```python
from build123d import *

# Parameters (mm, degrees)
SKETCH1_W           = 100
SKETCH1_H           = 6.794919243
BOSS_EXTRUDE1_DEPTH = 102.5
CIRPATTERN1_COUNT   = 4


with BuildPart() as part:
    # Sketch1 → Boss-Extrude1 (new, symmetric)
    with BuildSketch(Plane(origin=(0, 0, 0), x_dir=(0, 0, -1), z_dir=(1, 0, 0))):
        Polygon((-200, 0), (-100, 0), (-100, 6.794919243), (-100, 26.794919243), align=None)
        with Locations((-50, 3.397459622)):
            Rectangle(SKETCH1_W, SKETCH1_H)
    boss_extrude1 = extrude(amount=BOSS_EXTRUDE1_DEPTH, both=True)

    # CirPattern1: Boss-Extrude1 ×4 about axis
    cirpattern1_axis = Axis((0, 0, 0), (0, 1, 0))
    for i in range(1, CIRPATTERN1_COUNT):
        add(boss_extrude1.rotate(cirpattern1_axis, i * 360 / CIRPATTERN1_COUNT))


solid = part.part
```
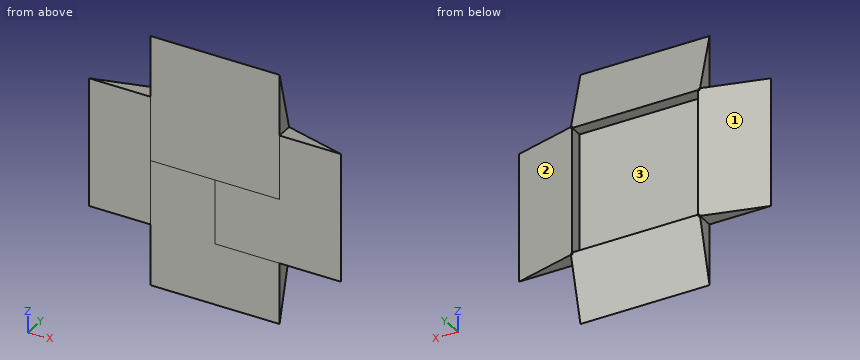
Could you check a few things on this model? Use its own coordinates, in mm. Face numbers are marked on the shaded views. Give positions to 0.01 mm unless a question says otherwise; leave off trailing zeros. Write each loop counter-clockwise with the first axis right and the second up, starting at its lowest first coordinate (ties: lowest second). Pieces come first, ordered by that corner, then holes. Notation, with made-up numbers: (8.25, 45) - (14.25, 45) arc R28 ccw to (14.25, 65) - close; hole circle Ø9 at (26.25, -3.5). An arc over 180 degrees is marked (long way). One line per item, written item: value. Start each with the question number.
Item 1: Imagine slicing it at D-D, the plane x = -152. List the corners of the cut face in (y, z) for me, and give its area (3 significant figures).
Item 2: I'm going to push flat-ended pins straight in: pin 1 (8 mm diameter, centred on x = -171, y = 15, fed in from -Z); pin 2 (5 mm diameter, centred on x = -115.5, y = 12.5, fed in from -Z); pin 3 (4 mm diameter, centred on x = 33.5, z = 80, fed in from +Y); pin 4 (13 mm diameter, centred on x = -145, y = 7.5, fed in from +Z). Where does each tip first touch, or does it pass through?
Item 3: Imagine slicing it at C-C, the plane y = 12.5. List the corners of the cut face in (x, z) for me, and give its area (3 significant figures).
Item 4: If we mould it in two halves opening along X, with no side actions, what happens to the marked faces 1, 2 and 3? For each: +X half, -X half, draft (parallel to the pull), parting line (faces both ways), or undercut.
Item 5: Imagine slicing it at A-A, the plane z = 76.5. List the corners of the cut face in (x, y) for me, and give its area (3 significant figures).
Item 6: Please list where these lines run through material, in increasing order: line 1 (Y direction, x = -47.5, z = 76.5); line 2 (X direction, y = 1, z = -141.5). Write a range as from..to.
Item 7: Imagine slicing it at B-B, the plane x = 54. List the corners of the cut face in (y, z) for me.
Geometry says:
1. outline: (0, -102.5) - (12.86, -102.5) - (12.86, 102.5) - (0, 102.5) - close
1. area: 2,640 mm^2
2. pin 1: through
2. pin 2: z = -102.5
2. pin 3: y = 6.79
2. pin 4: z = 102.5
3. outline: (-153.35, -102.5) - (-102.5, -102.5) - (-102.5, -153.35) - (102.5, -153.35) - (102.5, -102.5) - (153.35, -102.5) - (153.35, 102.5) - (102.5, 102.5) - (102.5, 153.35) - (-102.5, 153.35) - (-102.5, 102.5) - (-153.35, 102.5) - close; hole (-100, -100) - (100, -100) - (100, 100) - (-100, 100) - close
3. area: 43,700 mm^2
4. face 1: -X half
4. face 2: +X half
4. face 3: undercut
5. outline: (-200, 0) - (200, 0) - (100, 26.79) - (100, 6.79) - (-100, 6.79) - (-100, 26.79) - close
5. area: 4,040 mm^2
6. line 1: 0..6.79
6. line 2: -102.5..102.5
7. outline: (0, -200) - (26.79, -100) - (6.79, -100) - (6.79, 100) - (26.79, 100) - (0, 200) - close
